Read the model definition and answer for the solid it produces. Units are mm, in the model's axes. Face numbers are marked on the shaded views. A direction names the side the tool comes from. Coordinates: 2 decimals unless noted, no trailing zeros. Loops run counter-clockwise (first coordinate to the right, second up) from the corner with the lowest first, then second, coordinate; pieces in that order, holes last. Notation, with made-up numbers: M -1,80.25 L 10,80.25 A22 cw 10,103.25 Z; hole C 12.5,31 d6. An arc over 180 degrees is marked long. Use one line per item in the form item = value. Start each with the question number.
1. Find the intervals of material crossed by probe 1 along X at (y, z) = (61, 1); probe 2 along Z at (x, y) = (-27.15, 60); probe 3 along Z at (x, y) = (-13.5, 76.5), in increasing order. Write a range as [from, to].
2. The part is cut by section B-B (y = 62.75). Give the vertices of the cut face in (x, z), plus the area to 3 significant figures.
3. A tool of negligible diameter and unlimited length cuts with its end or side. For the marked faces 5, 6 and 7, from which of +Z, -Z, +X, -X, +Y, -Y can it reach the whole face along a straight path? Write none if from no direction.
4. The part is cut by section C-C (x = -16.5). Give the vertices of the cut face in (y, z).
5. The part is cut by section A-A (z = 2.5). Give the vertices of the cut face in (x, y), plus the area to 3 significant figures.
6. Flat-ended cylindrical pins translate along their axes: pin 1 (3 mm diameter, centred on x = -15, z = 2.5, fed in from -Y); pin 2 (1.5 mm diameter, centred on y = 80, z = 3, fed in from +X); pin 3 (1.5 mm diameter, centred on x = -14.5, z = 2, fed in from +Y). Find the tip coordinate at first contact, or state that the pin passes through.
7. For a pull along X with two mould halves and no side action, classify the marked faces 1, 2, 3 and 4 as released by +X, released by -X, zero draft, split by the parting line, or undercut.
8. The part is cut by section D-D (z = 4.5). Give the vertices of the cut face in (x, y).
from build123d import *
from build123d.topology import SkipClean

# Parameters (mm, degrees)
SKETCH1_W           = 20
SKETCH1_H           = 60
BOSS_EXTRUDE1_DEPTH = 5
SKETCH2_R           = 2.5
SKETCH2_R_2         = 1.25
BOSS_EXTRUDE2_DEPTH = 20
CUT_EXTRUDE1_START  = -29
SKETCH3_R           = 1.25
CUT_EXTRUDE1_DEPTH  = 29
SKETCH4_R           = 2.5
SKETCH4_R_2         = 1.25
BOSS_EXTRUDE3_DEPTH = 20
CUT_EXTRUDE2_START  = -29
SKETCH5_R           = 1.25
CUT_EXTRUDE2_DEPTH  = 29
SKETCH6_R           = 1.25
BOSS_EXTRUDE4_DEPTH = 30
SKETCH7_W           = 20.6
SKETCH7_H           = 7
CUT_EXTRUDE3_DEPTH  = 30
SKETCH8_W           = 60.511546569
SKETCH8_H           = 78.563917263
CUT_EXTRUDE4_DEPTH  = 41
SKETCH13_W          = 15
SKETCH13_H          = 15
BOSS_EXTRUDE6_DEPTH = 5
FILLET1_R           = 10
SKETCH14_W          = 5
SKETCH14_H          = 3
CUT_EXTRUDE6_DEPTH  = 14


with BuildPart() as part:
    # Sketch1 → Boss-Extrude1 (new body)
    with BuildSketch(Plane.XY):
        with Locations((10, 30)):
            Rectangle(SKETCH1_W, SKETCH1_H)
    extrude(amount=BOSS_EXTRUDE1_DEPTH)

    # Sketch2 → Boss-Extrude2 (add)
    with BuildSketch(Plane(origin=(20, 0, 0), x_dir=(0, 0, -1), z_dir=(1, 0, 0))):
        with Locations((-2.5, 60)):
            Circle(SKETCH2_R)
        with Locations((-2.5, 60)):
            Circle(SKETCH2_R_2, mode=Mode.SUBTRACT)
    extrude(amount=-BOSS_EXTRUDE2_DEPTH)

    # Sketch3 → Cut-Extrude1 (cut)
    with SkipClean():  # the faces are left unmerged after this step: merging them gives an invalid solid
        with BuildSketch(Plane.ZY.offset(CUT_EXTRUDE1_START)):
            with Locations(Location((2.5, 60, 0), (0, 0, 180))):
                Circle(SKETCH3_R)
        extrude(amount=CUT_EXTRUDE1_DEPTH, mode=Mode.SUBTRACT)

    # Sketch4 → Boss-Extrude3 (add)
    with BuildSketch(Plane.ZY):
        with Locations((2.5, 0)):
            Circle(SKETCH4_R)
        with Locations((2.5, 0)):
            Circle(SKETCH4_R_2, mode=Mode.SUBTRACT)
    extrude(amount=-BOSS_EXTRUDE3_DEPTH)

    # Sketch5 → Cut-Extrude2 (cut)
    with SkipClean():  # the faces are left unmerged after this step: merging them gives an invalid solid
        with BuildSketch(Plane(origin=(20, 0, 0), x_dir=(0, 0, -1), z_dir=(1, 0, 0)).offset(CUT_EXTRUDE2_START)):
            with Locations(Location((-2.5, 0, 0), (0, 0, 180))):
                Circle(SKETCH5_R)
        extrude(amount=CUT_EXTRUDE2_DEPTH, mode=Mode.SUBTRACT)

    # Sketch6 → Boss-Extrude4 (add)
    with SkipClean():  # the faces are left unmerged after this step: merging them gives an invalid solid
        with BuildSketch(Plane.ZY):
            with BuildLine():
                Line((5, 60), (5, 70))
                Line((5, 70), (0, 70))
                Line((0, 70), (0, 60))
                ThreePointArc((0, 60), (2.5, 57.5), (5, 60))
            make_face()
            with Locations(Location((2.5, 60, 0), (0, 0, 180))):
                Circle(SKETCH6_R, mode=Mode.SUBTRACT)
        extrude(amount=BOSS_EXTRUDE4_DEPTH)

    # Sketch7 → Cut-Extrude3 (cut)
    with SkipClean():  # the faces are left unmerged after this step: merging them gives an invalid solid
        with BuildSketch(Plane(origin=(0, 0, 0), x_dir=(-1, 0, 0), z_dir=(0, 0, -1))):
            with Locations((15, 60)):
                Rectangle(SKETCH7_W, SKETCH7_H)
        extrude(amount=-CUT_EXTRUDE3_DEPTH, mode=Mode.SUBTRACT)

    # Sketch8 → Cut-Extrude4 (cut)
    with BuildSketch(Plane.ZY):
        with Locations((2.066743104, 31.078249137)):
            Rectangle(SKETCH8_W, SKETCH8_H)
    extrude(amount=-CUT_EXTRUDE4_DEPTH, mode=Mode.SUBTRACT)

    # Sketch13 → Boss-Extrude6 (add)
    with BuildSketch(Plane(origin=(0, 0, 0), x_dir=(-1, 0, 0), z_dir=(0, 0, -1))):
        with Locations((15, 77.5)):
            Rectangle(SKETCH13_W, SKETCH13_H)
    extrude(amount=-BOSS_EXTRUDE6_DEPTH)

    # Fillet1
    # the kernel refuses this fillet: 10 mm, written as the material it adds along each edge
    with BuildSketch(Plane(origin=(-22.5, 70, 0), x_dir=(-1, 0, 0), z_dir=(0, 0, 1))) as fillet1_piece_1:
        with BuildLine():
            CenterArc((10, -9.682458366), FILLET1_R, 104.477512186, 75.522487814)
            Line((0, -9.682458366), (-0.2, -9.682458366))
            Line((-0.2, -9.682458366), (-0.2, 0))
            Line((-0.2, 0), (0, 0.2))
            ThreePointArc((0, 0.2), (3.75, 0.2), (7.45, 0.193649167))
            Line((7.45, 0.193649167), (7.5, 0))
        make_face()
    extrude(amount=5)
    with BuildSketch(Plane(origin=(-7.5, 70, 0), x_dir=(1, 0, 0), z_dir=(0, 0, 1))) as fillet1_piece_2:
        with BuildLine():
            CenterArc((10, 9.682458366), FILLET1_R, 180, 75.522487814)
            Line((0, 9.682458366), (-0.2, 9.682458366))
            Line((-0.2, 9.682458366), (-0.2, 0))
            Line((-0.2, 0), (0, -0.2))
            ThreePointArc((0, -0.2), (3.75, -0.2), (7.45, -0.193649167))
            Line((7.45, -0.193649167), (7.5, 0))
        make_face()
    extrude(amount=5)

    # Sketch14 → Cut-Extrude6 (cut)
    with BuildSketch(Plane(origin=(0, 85, 0), x_dir=(1, 0, 0), z_dir=(0, 1, 0))):
        with Locations((-15, -2.5)):
            Rectangle(SKETCH14_W, SKETCH14_H)
    extrude(amount=-CUT_EXTRUDE6_DEPTH, mode=Mode.SUBTRACT)


solid = part.part
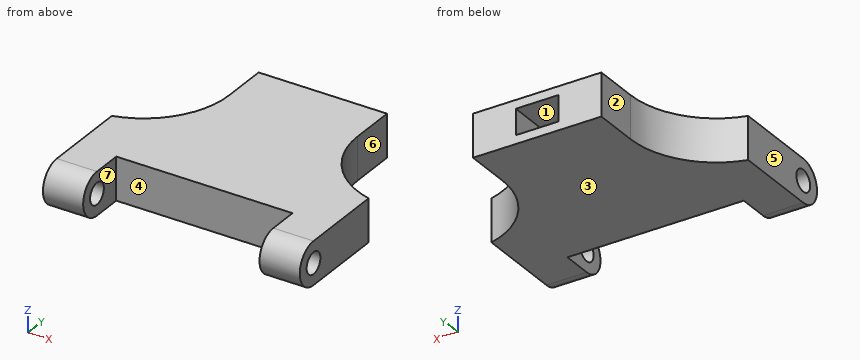
Computed values:
q1.probe_1 = [-30, -25.3], [-4.7, 0]
q1.probe_2 = [0, 1.25], [3.75, 5]
q1.probe_3 = [0, 1], [4, 5]
q2.outline = M -30,0 L -25.3,0 L -25.3,5 L -30,5 Z; M -4.7,0 L 0,0 L 0,5 L -4.7,5 Z
q2.area = 47.0 mm²
q3.face_5 = +Z, -Z, -X, +Y, -Y
q3.face_6 = +Z, -Z, +X, +Y
q3.face_7 = +Z, -Z, -Y
q4.outline = M 63.5,0 L 85,0 L 85,1 L 71,1 L 71,4 L 85,4 L 85,5 L 63.5,5 Z
q5.outline = M -30,57.5 L -25.3,57.5 L -25.3,58.75 L -30,58.75 Z; M -30,61.25 L -25.3,61.25 L -25.3,63.5 L -4.7,63.5 L -4.7,61.25 L 0,61.25 L 0,70 A10 cw -7.5,79.68 L -7.5,85 L -12.5,85 L -12.5,71 L -17.5,71 L -17.5,85 L -22.5,85 L -22.5,79.68 A10 cw -30,70 Z; M -4.7,57.5 L 0,57.5 L 0,58.75 L -4.7,58.75 Z
q5.area = 421 mm²
q6.pin_1 = 63.5
q6.pin_2 = -7.49
q6.pin_3 = 71
q7.face_1 = undercut
q7.face_2 = released by -X
q7.face_3 = zero draft
q7.face_4 = undercut
q8.outline = M -30,58.5 L -25.3,58.5 L -25.3,63.5 L -4.7,63.5 L -4.7,58.5 L 0,58.5 L 0,70 A10 cw -7.5,79.68 L -7.5,85 L -22.5,85 L -22.5,79.68 A10 cw -30,70 Z
